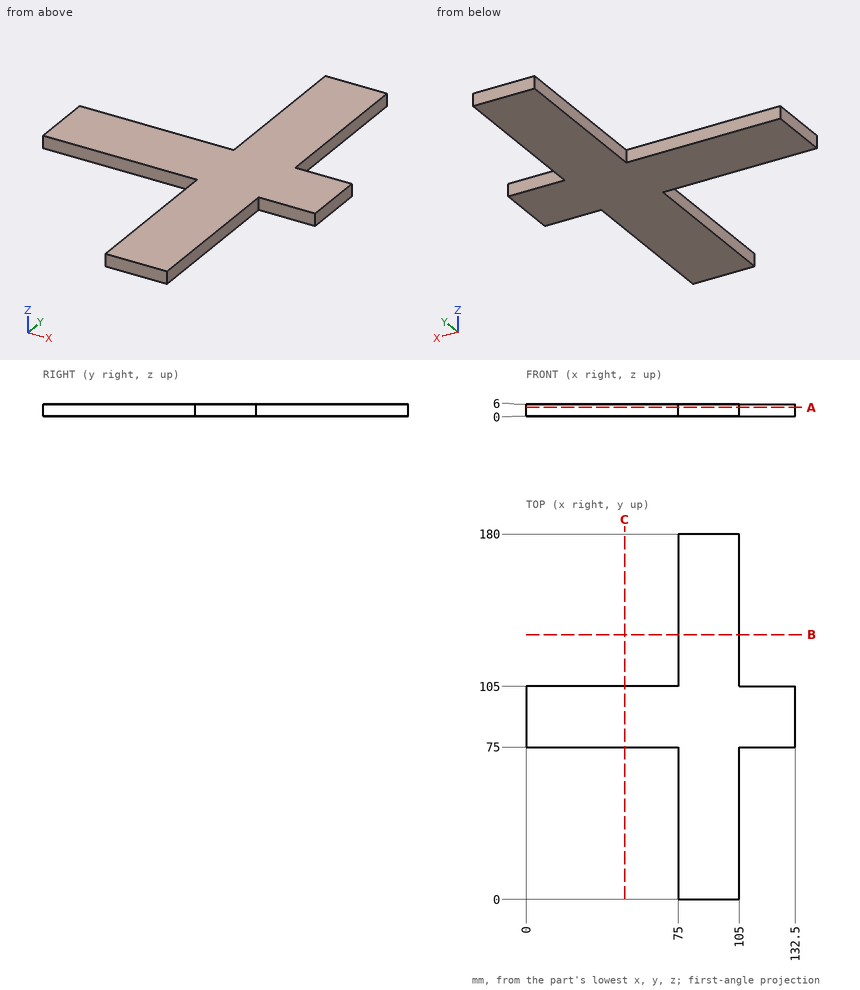
The figure shows three views and two pictorial views of one solid part (mm, origin at its lowest corner). Answer the questions. Give positions to 0.01 mm unless a question says otherwise; leave off trailing zeros. Loops run counter-clockwise (first coordinate to the right, second up) from the corner with the lowest first, then second, coordinate; pieces in that order, holes last. Notation, with made-up numbers: M -29,30.5 L 4,30.5 A15 ccw 4,54.5 Z; hole C 40,-12.5 d4. An arc over 180 degrees is marked long. Write each question's results on one line, items separated by ' | '.
1. A straight line is drawn through the part: line 1 (Y direction, x = 49, z = 0.8). Find the intervals that lie inside material, in ascending order. Write a range as [from, to].
Values:
line 1: y = [75, 105]
2. Section B-B on y = 130.5 is taken. Give the vertices of the cut face in (x, z), plus the area to 3 significant figures.
Values:
outline: M 75,0 L 105,0 L 105,6 L 75,6 Z | area: 180 mm^2
3. Section A-A on z = 4.3 is taken. Give the vertices of the cut face in (x, y), plus the area to 4 significant figures.
Values:
outline: M 0,75 L 75,75 L 75,0 L 105,0 L 105,75 L 132.5,75 L 132.5,105 L 105,105 L 105,180 L 75,180 L 75,105 L 0,105 Z | area: 8,475 mm^2
4. Given pin 1 (1.8 mm diameter, centred on y = 36.5, z = 2, fed in from -X); pin 2 (3 mm diameter, centred on x = 113, z = 4, fed in from +Y); pin 3 (3 mm diameter, centred on x = 108, z = 5, fed in from -Y), each flat-ended and moving along its own axis, determine where each tip first touches the part or whether it passes through.
Values:
pin 1: stops at x = 75 | pin 2: stops at y = 105 | pin 3: stops at y = 75
